from build123d import *

# Parameters (mm, degrees)
SKETCH1_W           = 100
SKETCH1_H           = 254
BOSS_EXTRUDE1_DEPTH = 3
SKETCH2_W           = 3
SKETCH2_H           = 35
SKETCH2_H_2         = 40
BOSS_EXTRUDE2_DEPTH = 3
SKETCH3_W           = 20
SKETCH3_H           = 3
CUT_EXTRUDE1_DEPTH  = 3
SKETCH4_W           = 20
SKETCH4_H           = 3
CUT_EXTRUDE2_DEPTH  = 3
SKETCH5_R           = 20
SKETCH5_R_2         = 10.25
SKETCH5_R_3         = 1.6
SKETCH5_R_4         = 14.25
SKETCH5_R_5         = 12.25
SKETCH5_R_6         = 2.6
SKETCH5_R_7         = 6
CUT_EXTRUDE3_DEPTH  = 3
SKETCH6_W           = 50
SKETCH6_H           = 3
BOSS_EXTRUDE3_DEPTH = 3
SKETCH8_W           = 3
SKETCH8_H           = 35
BOSS_EXTRUDE4_DEPTH = 3


with BuildPart() as part:
    # Sketch1 → Boss-Extrude1 (new body)
    with BuildSketch(Plane.XY):
        Rectangle(SKETCH1_W, SKETCH1_H)
    extrude(amount=BOSS_EXTRUDE1_DEPTH)

    # Sketch2 → Boss-Extrude2 (add)
    with BuildSketch(Plane(origin=(50, 0, 0), x_dir=(0, 0, -1), z_dir=(1, 0, 0))):
        with Locations((-1.5, 72.5)):
            Rectangle(SKETCH2_W, SKETCH2_H)
        with Locations((-1.5, 0)):
            Rectangle(SKETCH2_W, SKETCH2_H_2)
        with Locations((-1.5, -72.5)):
            Rectangle(SKETCH2_W, SKETCH2_H)
    extrude(amount=BOSS_EXTRUDE2_DEPTH)

    # Sketch3 → Cut-Extrude1 (cut)
    with BuildSketch(Plane(origin=(0, 127, 0), x_dir=(1, 0, 0), z_dir=(0, 1, 0))):
        with Locations((25, -1.5)):
            Rectangle(SKETCH3_W, SKETCH3_H)
        with Locations((-25, -1.5)):
            Rectangle(SKETCH3_W, SKETCH3_H)
    extrude(amount=-CUT_EXTRUDE1_DEPTH, mode=Mode.SUBTRACT)

    # Sketch4 → Cut-Extrude2 (cut)
    with BuildSketch(Plane.XY.offset(3)):
        with Locations((-25, -40.5)):
            Rectangle(SKETCH4_W, SKETCH4_H)
        with Locations((20, -40.5)):
            Rectangle(SKETCH4_W, SKETCH4_H)
    extrude(amount=-CUT_EXTRUDE2_DEPTH, mode=Mode.SUBTRACT)

    # Sketch5 → Cut-Extrude3 (cut)
    with BuildSketch(Plane.XY.offset(3)):
        with Locations((0, -88)):
            Circle(SKETCH5_R)
        with Locations((-25.5, 41.5)):
            Circle(SKETCH5_R_2)
        with Locations((-36.5, 52.5)):
            Circle(SKETCH5_R_3)
        with Locations((-14.5, 52.5)):
            Circle(SKETCH5_R_3)
        with Locations((-36.5, 30.5)):
            Circle(SKETCH5_R_3)
        with Locations((-14.5, 30.5)):
            Circle(SKETCH5_R_3)
        with Locations((-17, 6)):
            Circle(SKETCH5_R_3)
        with Locations((13, 6)):
            Circle(SKETCH5_R_3)
        with Locations((-17, -24)):
            Circle(SKETCH5_R_3)
        with Locations((13, -24)):
            Circle(SKETCH5_R_3)
        with Locations((-2, -9)):
            Circle(SKETCH5_R_4)
        with Locations((11, 40)):
            Circle(SKETCH5_R_5)
        with Locations((-2, 53)):
            Circle(SKETCH5_R_3)
        with Locations((24, 53)):
            Circle(SKETCH5_R_3)
        with Locations((24, 27)):
            Circle(SKETCH5_R_3)
        with Locations((-2, 27)):
            Circle(SKETCH5_R_3)
        with Locations(Location((-19.67760104, 94.560133375, 0), (0, 0, 180))):
            Circle(SKETCH5_R_6)
        with Locations(Location((-11.69545935, 75.136297141, 0), (0, 0, 180))):
            Circle(SKETCH5_R_6)
        with Locations(Location((12.69545935, 107.863702859, 0), (0, 0, 180))):
            Circle(SKETCH5_R_6)
        with Locations(Location((20.67760104, 88.439866625, 0), (0, 0, 180))):
            Circle(SKETCH5_R_6)
        with Locations((-34, 10)):
            Circle(SKETCH5_R_7)
        with Locations((-34, -22)):
            Circle(SKETCH5_R_7)
        with BuildLine():
            Line((8.003725129, 100.864513292), (0.511048213, 119.097280263))
            ThreePointArc((0.511048213, 119.097280263), (-0.28284909, 120.035570092), (-1.475557752, 120.33239795))
            ThreePointArc((-1.475557752, 120.33239795), (-10.484947373, 118.230898436), (-18.368690592, 113.3902379))
            ThreePointArc((-18.368690592, 113.3902379), (-19.008046594, 112.340530973), (-18.912788021, 111.115138573))
            Line((-18.912788021, 111.115138573), (-11.420111105, 92.882371602))
            ThreePointArc((-11.420111105, 92.882371602), (-10.599334991, 86.938776177), (-7.003725129, 82.135486708))
            Line((-7.003725129, 82.135486708), (0.488951787, 63.902719737))
            ThreePointArc((0.488951787, 63.902719737), (1.28284909, 62.964429908), (2.475557752, 62.66760205))
            ThreePointArc((2.475557752, 62.66760205), (11.484947373, 64.769101564), (19.368690592, 69.6097621))
            ThreePointArc((19.368690592, 69.6097621), (20.008046594, 70.659469027), (19.912788021, 71.884861427))
            Line((19.912788021, 71.884861427), (12.420111105, 90.117628398))
            ThreePointArc((12.420111105, 90.117628398), (11.599334991, 96.061223823), (8.003725129, 100.864513292))
        make_face()
    extrude(amount=-CUT_EXTRUDE3_DEPTH, mode=Mode.SUBTRACT)

    # Sketch6 → Boss-Extrude3 (add)
    with BuildSketch(Plane.XZ.offset(127)):
        with Locations((3, 1.5)):
            Rectangle(SKETCH6_W, SKETCH6_H)
    extrude(amount=BOSS_EXTRUDE3_DEPTH)

    # Sketch8 → Boss-Extrude4 (add)
    with BuildSketch(Plane.ZY.offset(50)):
        with Locations((1.5, -89.5)):
            Rectangle(SKETCH8_W, SKETCH8_H)
        with Locations((1.5, -4.5)):
            Rectangle(SKETCH8_W, SKETCH8_H)
        with Locations((1.5, 65.5)):
            Rectangle(SKETCH8_W, SKETCH8_H)
    extrude(amount=BOSS_EXTRUDE4_DEPTH)


solid = part.part
CAD build for the part. Positions are in the model's coordinates, mm. A direction names the side the tool comes from. Give positions to 0.01 mm unless a question says otherwise; leave off trailing zeros. Write each loop counter-clockwise with the first axis right and the second up, starting at its lowest first coordinate (ties: lowest second). Pieces come first, ordered by that corner, then holes. Notation, with made-up numbers: (15, -25) - (65, -25) arc R9 ccw to (65, -17) - close; hole circle Ø6 at (-18.75, -25.5). An arc over 180 degrees is marked (long way). Answer as CSV lines item,"result".
Q1. Band-saw the part on D-D (y = -65). Give the cut face in (x, z), and give its area (3 significant figures).
Result set:
outline,"(-50, 0) - (53, 0) - (53, 3) - (-50, 3) - close"
area,"309 mm²"
Q2. 3-axis set-ups, long thin cutter, end or side, ignore diameter. For faces 3 (the face through (-15.22, 102.13, 1.52)), 4 (the face through (11, 0, 3)): which of +Z, -Z, +X, -X, +Y, -Y reach the whole face in a straight line?
Result set:
face 3,"+Z, -Z"
face 4,"+Z, +X, -X, +Y, -Y"
Q3. Flat gauge pins, fed straight in: pin 1 Ø7 at (x, y) = (-34, 10) entering from +Z; pin 2 Ø0.9 at (y, z) = (-128, 1) entering from +X; pin 3 Ø3.5 at (x, y) = (-14.5, 52.5) entering from -Z; pin 4 Ø1.5 at (y, z) = (-128.5, 2) entering from -X. Where does each tip first touch, or does it go through?
Result set:
pin 1,"through"
pin 2,"x = 28"
pin 3,"z = 0"
pin 4,"x = -22"
Q4. Band-saw the part on C-C (z = 1.7). State how many separate pieces and enclosed holes the cut face has, and give its area (3 significant figures).
Result set:
separate pieces,"1"
enclosed holes,"25"
area,"21,600 mm²"
Q5. Band-saw the part on A-A (x = -25.5). Give the cut face in (y, z).
Result set:
outline,"(-127, 0) - (-42, 0) - (-42, 3) - (-127, 3) - close; (-39, 0) - (31.25, 0) - (31.25, 3) - (-39, 3) - close; (51.75, 0) - (124, 0) - (124, 3) - (51.75, 3) - close"
Q6. Pull direction Y, two halves, no side cores. Call faces 1 (the face through (11, 0, 0)), 2 (the face through (15.293, 107.749, 1.521)): released by +Y, released by -Y, zero draft, split by the parting line, or undercut.
Result set:
face 1,"zero draft"
face 2,"undercut"
Q7. Drill centre lines: line 1 (Y direction, x = -9, z = 2.2); line 2 (Y direction, x = 3, z = 1.15); line 3 (Y direction, x = -2, z = 1.5). Where is each one in solid material? Low to high. Write a range as from..to.
Result set:
line 1,"-130..-105.86, -70.14..-21.41, 3.41..84.17, 118.79..127"
line 2,"-130..-107.77, -68.23..-22.34, 4.34..30.72, 49.28..62.71, 113.04..127"
line 3,"-130..-107.9, -68.1..-23.25, 5.25..25.4, 28.6..51.4, 54.6..69.96, 120.29..127"
Q8. Band-saw the part on B-B (y = 10). Give the cut face in (x, z).
Result set:
outline,"(-53, 0) - (-40, 0) - (-40, 3) - (-53, 3) - close; (-28, 0) - (53, 0) - (53, 3) - (-28, 3) - close"
